For this review, use the dimensioned drawing (mm, ordinates from the lowest corner) and the shaded views. A direction names the side the tool comes from. Coordinates: 2 decimals unless noted, no trailing zeros. Write each loop counter-clockwise with the first axis right and the second up, starting at its lowest first coordinate (ties: lowest second). Pieces come first, ordered by that corner, then holes. Notation, with made-up numbers: (18, 14.5) -> (54, 14.5) arc R21 cw to (54, 38.5) -> close; hole circle Ø7 at (-28, 68.25). An arc over 180 degrees is marked (long way). Put each result on its own line as item: value. Start each with the question number.
Item 1: Consider section D-D on y = 43.5. Give the boundary of the cut face in (x, z).
Item 2: Consider section C-C on x = 168. Give the boundary of the cut face in (y, z), and give its area (3 significant figures).
Item 3: Consider section B-B on z = 93. Give the boundary of the cut face in (x, y).
Item 4: Consider section A-A on y = 164. Give the boundary of the cut face in (x, z).
Item 5: To check wall thickness, follow L1, parallel to X at y = 64.5, z = 56.5; L2, parallel to X at y = 58.5, z = 62.5 (1 decimal); L3, parallel to Y at x = 106, z = 217.5. State the ranges of each line that lie inside material, in increasing order.
Item 6: For the marked faces 1 and 2, list the 3-axis set-ups (+Z, -Z, +X, -X, +Y, -Y) from which the entire face can be reached by the end or side of a thin tool; tool diameter is ignored.
Item 7: Insertion check: P1, Ø6, axis at x = 169, y = 132, coming from the +Z side; P2, Ø12, axis at x = 206, y = 123.5, coming from the +Z side; P3, Ø1.5, axis at x = 146, y = 120.5, coming from the -Z side. Each pin has a flat end and moves straight along its axis. Give the tip position at first contact, or say it passes through.
Item 8: The part is to be moulded in two halves that separate along X. For the marked faces 3, 4 and 5, say which applies: +X half, -X half, draft (parallel to the pull), parting line (faces both ways), or undercut.
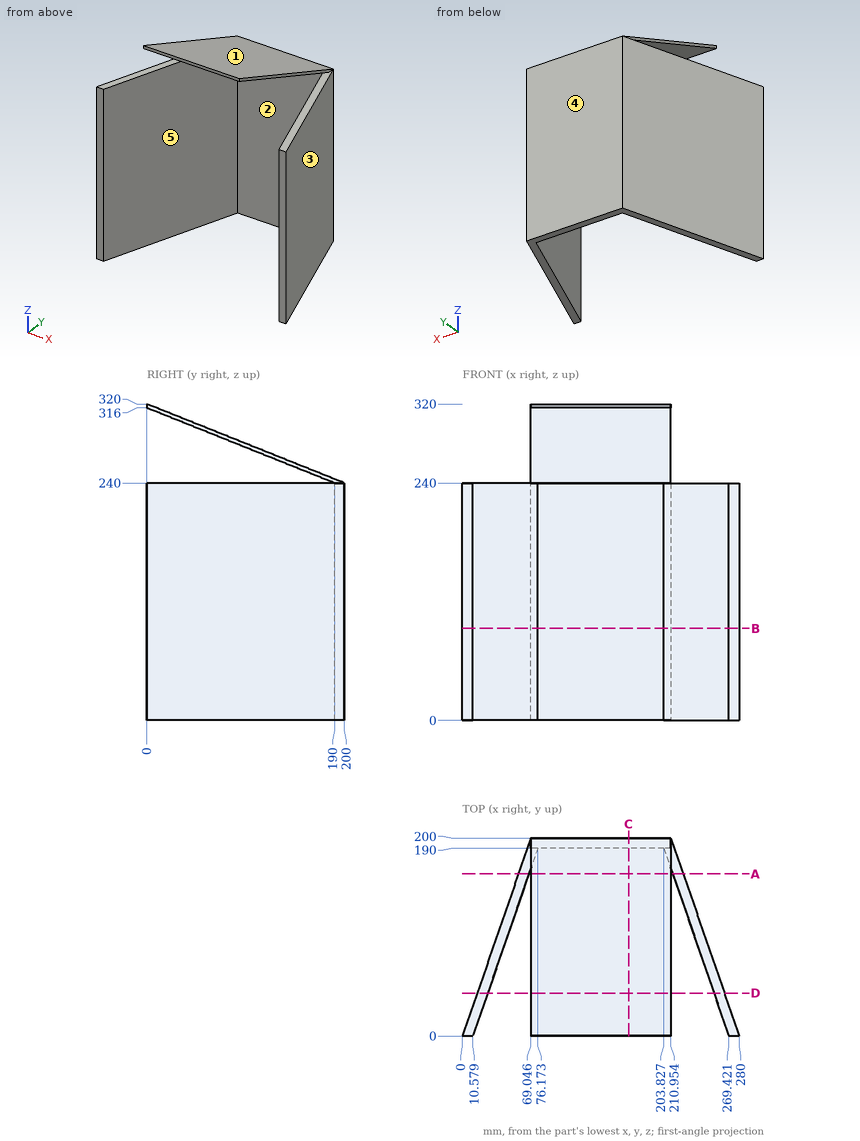
Return value:
1. outline: (15.02, 0) -> (25.6, 0) -> (25.6, 240) -> (15.02, 240) -> close; (69.05, 298.6) -> (210.95, 298.6) -> (210.95, 302.6) -> (69.05, 302.6) -> close; (254.4, 0) -> (264.98, 0) -> (264.98, 240) -> (254.4, 240) -> close
2. outline: (0, 316) -> (190, 240) -> (190, 0) -> (200, 0) -> (200, 240) -> (0, 320) -> close
2. area: 3,180 mm^2
3. outline: (0, 0) -> (10.58, 0) -> (76.17, 190) -> (203.83, 190) -> (269.42, 0) -> (280, 0) -> (210.95, 200) -> (69.05, 200) -> close
4. outline: (56.62, 0) -> (67.2, 0) -> (67.2, 240) -> (56.62, 240) -> close; (69.05, 250.4) -> (210.95, 250.4) -> (210.95, 254.4) -> (69.05, 254.4) -> close; (212.8, 0) -> (223.38, 0) -> (223.38, 240) -> (212.8, 240) -> close
5. L1: 22.27 to 32.85, 247.15 to 257.73
5. L2: 20.2 to 30.8, 249.2 to 259.8
5. L3: 190 to 200
6. face 1: +Z, +X, -X, +Y
6. face 2: -Z, -Y
7. P1: z = 268.4
7. P2: z = 273
7. P3: z = 267.5
8. face 3: +X half
8. face 4: draft
8. face 5: undercut
